from build123d import *

# Parameters (mm, degrees)
SZKIC1_W                    = 7
SZKIC1_H                    = 14.6
DODANIE_WYCI_GNI_CIE1_DEPTH = 8
SZKIC2_W                    = 2
SZKIC2_H                    = 5
WYTNIJ_WYCI_GNI_CIE1_DEPTH  = 3.5
SZKIC7_R                    = 3.25
SZKIC7_R_2                  = 2.25
WYTNIJ_WYCI_GNI_CIE4_DEPTH  = 3.8
SZKIC10_W                   = 2
SZKIC10_H                   = 6.184658438
WYTNIJ_WYCI_GNI_CIE6_DEPTH  = 3.8
SZKIC12_W                   = 1.5
SZKIC12_H                   = 2
DODANIE_WYCI_GNI_CIE4_DEPTH = 2
SZKIC15_W                   = 2.5
SZKIC15_H                   = 4.8
DODANIE_WYCI_GNI_CIE6_DEPTH = 1.2
SZKIC16_W                   = 2
SZKIC16_H                   = 1
DODANIE_WYCI_GNI_CIE7_DEPTH = 1
ZAOKR_GLENIE2_R             = 1
SZKIC17_W                   = 2
SZKIC17_H                   = 3.8
WYTNIJ_WYCI_GNI_CIE7_DEPTH  = 2


with BuildPart() as part:
    # Szkic1 → Dodanie-wyciągnięcie1 (new body)
    with BuildSketch(Plane(origin=(0, 0, 0), x_dir=(1, 0, 0), z_dir=(0, 1, 0))):
        with Locations((3.5, 7.3)):
            Rectangle(SZKIC1_W, SZKIC1_H)
    extrude(amount=DODANIE_WYCI_GNI_CIE1_DEPTH)

    # Szkic2 → Wytnij-wyciągnięcie1 (cut)
    with BuildSketch(Plane.XZ):
        with Locations((3.5, -7.3)):
            Rectangle(SZKIC2_W, SZKIC2_H)
    extrude(amount=-WYTNIJ_WYCI_GNI_CIE1_DEPTH, mode=Mode.SUBTRACT)

    # Szkic7 → Wytnij-wyciągnięcie4 (cut)
    with BuildSketch(Plane.XY):
        with Locations((3.5, 4)):
            Circle(SZKIC7_R)
        with Locations((3.5, 4)):
            Circle(SZKIC7_R_2, mode=Mode.SUBTRACT)
    extrude(amount=-WYTNIJ_WYCI_GNI_CIE4_DEPTH, mode=Mode.SUBTRACT)

    # Szkic10 → Wytnij-wyciągnięcie6 (cut)
    with BuildSketch(Plane.XY):
        with Locations((3.5, 4)):
            Rectangle(SZKIC10_W, SZKIC10_H)
    extrude(amount=-WYTNIJ_WYCI_GNI_CIE6_DEPTH, mode=Mode.SUBTRACT)

    # Szkic12 → Dodanie-wyciągnięcie4 (add)
    with BuildSketch(Plane(origin=(2.5, 0, 0), x_dir=(0, 0, -1), z_dir=(1, 0, 0))):
        with Locations((0.75, 4)):
            Rectangle(SZKIC12_W, SZKIC12_H)
    extrude(amount=DODANIE_WYCI_GNI_CIE4_DEPTH)

    # Szkic15 → Dodanie-wyciągnięcie6 (add)
    with BuildSketch(Plane.XZ):
        with Locations((3.5, -2.4)):
            Rectangle(SZKIC15_W, SZKIC15_H)
        with Locations((3.5, -12.2)):
            Rectangle(SZKIC15_W, SZKIC15_H)
    extrude(amount=DODANIE_WYCI_GNI_CIE6_DEPTH)

    # Szkic16 → Dodanie-wyciągnięcie7 (add)
    with BuildSketch(Plane.XZ.offset(-3.5)):
        with Locations((3.5, -7.3)):
            Rectangle(SZKIC16_W, SZKIC16_H)
    extrude(amount=DODANIE_WYCI_GNI_CIE7_DEPTH)

    # Zaokrąglenie2
    zaokr_glenie2_edges = [part.edges().sort_by_distance(p)[0] for p in [
        (3.5, -1.2, -14.6),
        (3.5, -1.2, 0),
    ]]
    fillet(zaokr_glenie2_edges, radius=ZAOKR_GLENIE2_R)

    # Szkic17 → Wytnij-wyciągnięcie7 (cut)
    with BuildSketch(Plane(origin=(0, 8, 0), x_dir=(1, 0, 0), z_dir=(0, 1, 0))):
        with Locations((3.5, 1.9)):
            Rectangle(SZKIC17_W, SZKIC17_H)
    extrude(amount=-WYTNIJ_WYCI_GNI_CIE7_DEPTH, mode=Mode.SUBTRACT)


solid = part.part
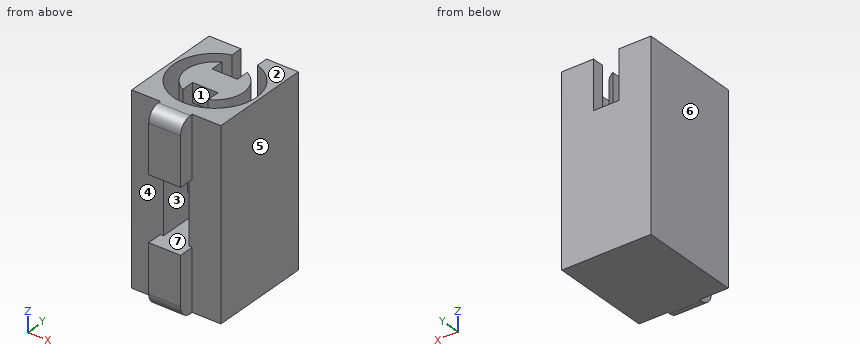
Input: part model. Units: mm. Frame: model coordinates. Face numbers are marked on the shaded views. A direction names the side the tool comes from. Round coordinates to 2 decimals unless told otherwise and drop trailing zeros. Order: outer loops, then holes, each group sorted by start corner. A loop starts at its lowest first (then second) coordinate and runs counter-clockwise, first axis right, second up. Notation, with made-up numbers: (-1.75, 46.25) - (40.25, 46.25) arc R22 cw to (40.25, 52.25) - close; hole circle Ø11 at (-12.5, 81.25). An arc over 180 degrees is marked (long way). Answer as a JSON object with one key per item and string values. Group by question number.
(1) Cut plane D-D (z = -10.75). Return loops of the section in (x, y), then the cut area to 3 significant figures.
(2) Draft query along X for the marked faces 4, 5, 6 and 7. Return one class per face: released by +X, released by -X, zero draft, split by the parting line, or undercut.
(3) Cut plane B-B (x = 3.5). Return loops of the section in (y, z), then the cut area to 3 significant figures.
(4) Material intervals for probe 1 along X at (y, z) = (4, -1.9); probe 2 along X at (y, z) = (4, -0.75); probe 3 along Y at (x, z) = (3.5, -1.3), sorted ascending. Write a range as from..to.
(5) Reachability of the marked faces 1, 2 and 3 from +Z, -Z, +X, -X, +Y, -Y: full face, straight path, thin tool, end or side. Return the list, or none.
(6) Cut plane A-A (y = 4). Return loops of the section in (x, z).
(7) Pin query (flat end, axial travel): P1, Ø0.8, axis at x = 3.5, z = -7, coming from the -Y side; P2, Ø1, axis at x = 3.5, z = -5.5, coming from the -Y side; P3, Ø1.2, axis at x = 3.5, z = -0.5, coming from the +Y side. Return the tip coordinate at first contact, or that it passes through.
(8) Cut plane C-C (z = -2.5). Return loops of the section in (x, y), then the cut area to 3 significant figures.
Here are the results:
{
 "1": {"outline": "(0, 0) - (2.25, 0) - (2.25, -1.2) - (4.75, -1.2) - (4.75, 0) - (7, 0) - (7, 8) - (0, 8) - close", "area": "59.0 mm^2"},
 "2": {"face 4": "zero draft", "face 5": "released by +X", "face 6": "released by -X", "face 7": "undercut"},
 "3": {"outline": "(-1.2, -13.6) arc R1 ccw to (-0.2, -14.6) - (8, -14.6) - (8, -3.8) - (0.75, -3.8) - (0.75, 0) - (-0.2, 0) arc R1 ccw to (-1.2, -1) - (-1.2, -4.8) - (3.5, -4.8) - (3.5, -6.8) - (2.5, -6.8) - (2.5, -7.8) - (3.5, -7.8) - (3.5, -9.8) - (-1.2, -9.8) - close; (3, -1.5) - (5, -1.5) - (5, 0) - (3, 0) - close", "area": "86.8 mm^2"},
 "4": {"probe 1": "x = 0..0.25, 1.25..2.5, 4.5..5.75, 6.75..7", "probe 2": "x = 0..0.25, 1.25..5.75, 6.75..7", "probe 3": "y = -1.2..0.75, 3..5"},
 "5": {"face 1": "+Z", "face 2": "+Z, +X, -X, +Y, -Y", "face 3": "-Y"},
 "6": {"outline": "(0, -14.6) - (7, -14.6) - (7, 0) - (6.75, 0) - (6.75, -3.8) - (5.75, -3.8) - (5.75, 0) - (1.25, 0) - (1.25, -3.8) - (0.25, -3.8) - (0.25, 0) - (0, 0) - close; hole (2.5, -3.8) - (4.5, -3.8) - (4.5, -1.5) - (2.5, -1.5) - close"},
 "7": {"P1": "stops at y = 2.5", "P2": "stops at y = 3.5", "P3": "stops at y = 5"},
 "8": {"outline": "(0, 0) - (2.25, 0) - (2.25, -1.2) - (4.75, -1.2) - (4.75, 0) - (7, 0) - (7, 8) - (4.5, 8) - (4.5, 7.09) arc R3.25 cw (long way) to (2.5, 7.09) - (2.5, 8) - (0, 8) - close; (2.5, 1.98) - (2.5, 6.02) arc R2.25 ccw to start; (4.5, 1.98) arc R2.25 ccw to (4.5, 6.02) - close", "area": "31.4 mm^2"}
}
